Read the model definition and answer for the solid it produces. Units are mm, in the model's axes. Coordinates: 2 decimals unless noted, no trailing zeros. Loops run counter-clockwise (first coordinate to the right, second up) from the corner with the lowest first, then second, coordinate; pieces in that order, holes last. Notation, with made-up numbers: (37, 1.25) -> (85, 1.25) arc R18 cw to (85, 19.25) -> close; hole circle Ø7 at (-1, -1.75). An arc over 180 degrees is marked (long way). Answer as a JSON object with one key per item and string values. Group by question number.
1) Consider probe 1 along X at (y, z) = (-5, -12); probe 2 along Z at (x, y) = (-393, 1); probe 3 along X at (y, z) = (1.5, -10). Determine where each line is inside the solid, lowest interval first. Write a range as [from, to].
2) Section C-C, the plane y = -11.5 is taken. Give the vertices of the cut face in (x, z).
3) Determine the mould class of faces 1 (the face through (6, 19.05, -1)), 2 (the face through (444.5, 0, 1)), 3 (the face through (383.6, -0.3, -20.4)) for opening direction X: released by +X, released by -X, zero draft, split by the parting line, or undercut.
4) Section D-D, the plane x = 277 is taken. Give the vertices of the cut face in (y, z).
5) Section B-B, the plane z = -12.7 is taken. Give the vertices of the cut face in (x, y).
6) Section A-A, the plane x = 393.7 is taken. Give the vertices of the cut face in (y, z), plus the area to 3 significant figures.
from build123d import *

# Parameters (mm, degrees)
F0_W     = 19.05
F0_H     = 139.7
F1_DEPTH = 444.5
F2_SIZE  = 19.05
F3_R     = 12.7
F4_DEPTH = 38.101


with BuildPart() as f1:
    # F0 (on Right) → F1 (new body, symmetric)
    with BuildSketch(Plane.YZ):
        with Locations((-9.525, 0)):
            Rectangle(F0_W, F0_H)
        with Locations((9.525, 0)):
            Rectangle(F0_W, F0_H)
    extrude(amount=F1_DEPTH, both=True)

    # F2
    f2_edges = [f1.edges().sort_by_distance(p)[0] for p in [
        (0, -19.05, 69.85),
    ]]
    chamfer(f2_edges, length=F2_SIZE)

    # F3 (on face) → F4 (cut, through all)
    with BuildSketch(Plane.XZ.offset(19.05)):
        with Locations((-393.7, -12.7)):
            Circle(F3_R)
        with Locations((393.7, -12.7)):
            Circle(F3_R)
    extrude(amount=-F4_DEPTH, mode=Mode.SUBTRACT)


solid = f1.part
Determined:
{
 "1": {"probe 1": "[-444.5, -406.38], [-381.02, 381.02], [406.38, 444.5]", "probe 2": "[-69.85, -25.38], [-0.02, 69.85]", "probe 3": "[-444.5, -406.11], [-381.29, 381.29], [406.11, 444.5]"},
 "2": {"outline": "(-444.5, -69.85) -> (444.5, -69.85) -> (444.5, 58.35) -> (-444.5, 58.35) -> close; hole circle Ø25.4 at (-393.7, -12.7); hole circle Ø25.4 at (393.7, -12.7)"},
 "3": {"face 1": "zero draft", "face 2": "released by +X", "face 3": "undercut"},
 "4": {"outline": "(-19.05, -69.85) -> (19.05, -69.85) -> (19.05, 69.85) -> (0, 69.85) -> (-19.05, 50.8) -> close"},
 "5": {"outline": "(-444.5, -19.05) -> (-406.4, -19.05) -> (-406.4, 19.05) -> (-444.5, 19.05) -> close; (-381, -19.05) -> (381, -19.05) -> (381, 19.05) -> (-381, 19.05) -> close; (406.4, -19.05) -> (444.5, -19.05) -> (444.5, 19.05) -> (406.4, 19.05) -> close"},
 "6": {"outline": "(-19.05, -69.85) -> (19.05, -69.85) -> (19.05, -25.4) -> (-19.05, -25.4) -> close; (-19.05, 0) -> (19.05, 0) -> (19.05, 69.85) -> (0, 69.85) -> (-19.05, 50.8) -> close", "area": "4,170 mm²"}
}
